```python
from build123d import *

# Parameters (mm, degrees)
CYLINDER_R       = 1.5
CYLINDER_DEPTH   = 10
EXTRUDE001_DEPTH = 2
EXTRUDE_DEPTH    = 5
CHAMFER_SIZE     = 0.45
CHAMFER001_SIZE  = 1.5


with BuildPart() as cylinder:
    # Cylinder → Cylinder (new body)
    with BuildSketch(Plane.XY.offset(-2)):
        Circle(CYLINDER_R)
    extrude(amount=CYLINDER_DEPTH)


with BuildPart() as extrude001:
    # Sketch001 → Extrude001 (new body)
    with BuildSketch(Plane.XY):
        with BuildLine():
            ThreePointArc((3.5, 13.5), (0, 17), (-3.5, 13.5))
            Line((-3.5, 13.5), (-3.5, 8.5))
            ThreePointArc((-3.5, 8.5), (0, 5), (3.5, 8.5))
            Line((3.5, 13.5), (3.5, 8.5))
        make_face()
    extrude(amount=EXTRUDE001_DEPTH)


with BuildPart() as obj1:
    # Sketch → Extrude (new body)
    with BuildSketch(Plane.XY):
        with BuildLine():
            Line((-5, 11), (-5, 0))
            ThreePointArc((-5, 0), (0, -5), (5, 0))
            Line((5, 11), (5, 0))
            ThreePointArc((5, 11), (3.5, 12.5), (2, 11))
            Line((2, 11), (2, 7.5))
            ThreePointArc((-2, 7.5), (0, 5.5), (2, 7.5))
            Line((-2, 11), (-2, 7.5))
            ThreePointArc((-2, 11), (-3.5, 12.5), (-5, 11))
        make_face()
    extrude(amount=EXTRUDE_DEPTH)

    # Cut: cut Extrude001
    add(extrude001.part, mode=Mode.SUBTRACT)

    # Chamfer
    chamfer_edges = [obj1.edges().sort_by_distance(p)[0] for p in [
        (-2.43934, 12.06066, 2),
        (-2, 9.25, 2),
        (2, 9.25, 2),
        (2.43934, 12.06066, 2),
    ]]
    chamfer(chamfer_edges, length=CHAMFER_SIZE)

    # Cut001: cut Cylinder
    add(cylinder.part, mode=Mode.SUBTRACT)

    # Chamfer001
    chamfer001_edges = [obj1.edges().sort_by_distance(p)[0] for p in [
        (-1.5, 0, 5),
    ]]
    chamfer(chamfer001_edges, length=CHAMFER001_SIZE)


solid = obj1.part
```
Source: CAD feature listing. Evaluate the final solid. Frame: model axes, mm. A direction names the side the tool comes from. Round coordinates to 2 decimals unless told otherwise and drop trailing zeros. Write each loop counter-clockwise with the first axis right and the second up, starting at its lowest first coordinate (ties: lowest second). Pieces come first, ordered by that corner, then holes. Notation, with made-up numbers: M 64.25,-39.75 L 108.25,-39.75 A25 cw 108.25,-25.75 Z; hole C 8,81.5 d6. An arc over 180 degrees is marked long. Use CSV: the item, a comma, the result in double quotes. Start each with the question number.
Q1. Pull-direction query (X, two-part tool) for faces 4 (the face through (-3.5, 11, 1)), 5 (the face through (5, 6, 2)), 6 (the face through (0, 2, 0)); classes: +X half, -X half, draft (parallel to the pull), parting line (faces both ways), or undercut.
Q2. First-contact query: P1, Ø5.5, axis at x = 1, y = 8, coming from the -Z side. Flat tip, straight axial feed; report the tip coordinate or a pass-through.
Q3. Cut plane B-B on z = 1.1. Output: boundary loops of the cut face in (x, y), plus the area to 3 significant figures.
Q4. Access query for faces 1 (the face through (0, 2, 4)), 2 (the face through (-3, 9, 2)), 3 (the face through (-2, 9, 4)). Directions: +Z, -Z, +X, -X, +Y, -Y. A direction counts if a zero-diameter tool reaches every point of the face in a straight line with its end or side. Return the directions, or none.
Q5. Line query: line 1 (X direction, y = 8, z = 4.4); line 2 (X direction, y = 0, z = 1.75); line 3 (Y direction, x = -1, z = 4.5). Output: solid intervals per line, ascending. Write a range as from..to.
Q6. Cut plane C-C on z = 4.45. Output: boundary loops of the cut face in (x, y).
Q7. Cut plane D-D on x = -4. Output: boundary loops of the cut face in (y, z), plus the area to 3 significant figures.
Q8. Cut plane A-A on x = 0. Output: boundary loops of the cut face in (y, z), plus the area to 3 significant figures.
Results found:
1,face 4,"undercut"
1,face 5,"+X half"
1,face 6,"draft"
2,P1,"z = 0"
3,outline,"M -5,0 A5 ccw 5,0 L 5,11 A1.5 ccw 3.5,12.5 L 3.5,8.5 A3.5 cw -3.5,8.5 L -3.5,12.5 A1.5 ccw -5,11 Z; hole C 0,0 d3"
3,area,"109 mm^2"
4,face 1,"+Z"
4,face 2,"-Z, +Y"
4,face 3,"+Z, -Z, +Y"
5,line 1,"-5..-2, 2..5"
5,line 2,"-5..-1.5, 1.5..5"
5,line 3,"-4.9..-2.29, 2.29..5.77"
6,outline,"M -5,0 A5 ccw 5,0 L 5,11 A1.5 ccw 2,11 L 2,7.5 A2 cw -2,7.5 L -2,11 A1.5 ccw -5,11 Z; hole C 0,0 d4.9"
7,outline,"M -3,0 L 12.41,0 L 12.41,5 L -3,5 Z"
7,area,"77.1 mm^2"
8,outline,"M -5,0 L -1.5,0 L -1.5,3.5 L -3,5 L -5,5 Z; M 1.5,0 L 5,0 L 5,2 L 5.05,2 L 5.5,2.45 L 5.5,5 L 3,5 L 1.5,3.5 Z"
8,area,"34.1 mm^2"
